Read the model definition and answer for the solid it produces. Units are mm, in the model's axes. Round coordinates to 2 decimals unless told otherwise and drop trailing zeros. Write each loop counter-clockwise with the first axis right and the second up, starting at its lowest first coordinate (ties: lowest second). Pieces come first, ordered by that corner, then holes. Notation, with made-up numbers: (-1.5, 44) - (52.5, 44) arc R11 cw to (52.5, 56) - close; hole circle Ø9 at (-7, 11.5). An arc over 180 degrees is marked (long way). Answer as CSV lines item,"result". Start each with the question number.
1) Find section B-B on z = 38.5. Determine the outline of the cut face in (x, y), then the cut area to 3 significant figures.
2) Find section C-C on y = 0. Determine the outline of the cut face in (x, z).
3) Find section D-D on x = -1.75. Determine the outline of the cut face in (y, z), then the cut area to 3 significant figures.
4) Find section A-A on x = -4. Determine the outline of the cut face in (y, z), then the cut area to 3 significant figures.
5) Each of these flat-tipped pins is pushed along its axis until it touches: pin 1 (1.2 mm diameter, centred on y = -1, z = 52, fed in from -X); pin 2 (2 mm diameter, centred on y = 2.5, z = 53, fed in from +X). Where does it stop, or does it pass through?
6) Consider line 1 along Z through (x, y) = (-1.3, 0); line 2 along Z through (x, y) = (-2.9, 0); line 3 along X through (y, z) = (0, 35). Determine where each line is inside the solid, lowest interval first.
from build123d import *

# Parameters (mm, degrees)
SKETCH1_R           = 5
BOSS_EXTRUDE1_DEPTH = 60
SKETCH2_W           = 5
SKETCH2_H           = 4
CUT_EXTRUDE1_DEPTH  = 40
SKETCH4_R           = 2
CUT_EXTRUDE2_DEPTH  = 40


with BuildPart() as part:
    # Sketch1 → Boss-Extrude1 (new body)
    with BuildSketch(Plane.XY):
        Circle(SKETCH1_R)
    extrude(amount=BOSS_EXTRUDE1_DEPTH)

    # Sketch2 → Cut-Extrude1 (cut)
    with BuildSketch(Plane(origin=(0, 0, 0), x_dir=(-1, 0, 0), z_dir=(0, 0, -1))):
        Rectangle(SKETCH2_W, SKETCH2_H)
    extrude(amount=-CUT_EXTRUDE1_DEPTH, mode=Mode.SUBTRACT)

    # Sketch4 → Cut-Extrude2 (cut)
    with BuildSketch(Plane(origin=(0, 0, 0), x_dir=(0, 0, -1), z_dir=(1, 0, 0))):
        with Locations((-52, 0)):
            Circle(SKETCH4_R)
    extrude(amount=-CUT_EXTRUDE2_DEPTH, mode=Mode.SUBTRACT)


solid = part.part
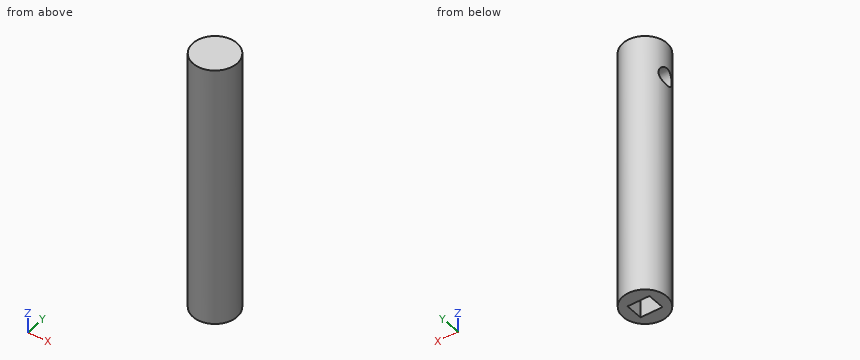
Check values:
1,outline,"circle Ø10 at (0, 0); hole (-2.5, -2) - (2.5, -2) - (2.5, 2) - (-2.5, 2) - close"
1,area,"58.5 mm^2"
2,outline,"(-5, 0) - (-2.5, 0) - (-2.5, 40) - (2.5, 40) - (2.5, 0) - (5, 0) - (5, 60) - (-5, 60) - (-5, 54) - (0, 54) - (0, 50) - (-5, 50) - close"
3,outline,"(-4.68, 0) - (-2, 0) - (-2, 40) - (2, 40) - (2, 0) - (4.68, 0) - (4.68, 60) - (-4.68, 60) - close; hole circle Ø4 at (0, 52)"
3,area,"389 mm^2"
4,outline,"(-3, 0) - (3, 0) - (3, 60) - (-3, 60) - close; hole circle Ø4 at (0, 52)"
4,area,"347 mm^2"
5,pin 1,"stops at x = 0"
5,pin 2,"stops at x = 4.77"
6,line 1,"z = 40 to 50, 54 to 60"
6,line 2,"z = 0 to 50, 54 to 60"
6,line 3,"x = -5 to -2.5, 2.5 to 5"
